```python
from build123d import *

# Parameters (mm, degrees)
HOLE_D             = 4.5
HOLE_DEPTH         = 25
HOLE_CSINK_D       = 9.5
HOLE_CSINK_ANGLE   = 90
POLARPATTERN_COUNT = 6
SKETCH002_W        = 110
SKETCH002_H        = 70.917771
POCKET_DEPTH       = 41.103131
POCKET_DEPTH_BACK  = -41.103131


with BuildPart() as part:
    # Sketch → Revolution (revolve)
    with BuildSketch(Plane.XZ):
        Polygon((-27.5, 18), (-27.5, 0), (-25.5, 0), (-25.5, 40), (-27.5, 45), (-27.5, 25), (-30.5, 22), (-41.102131, 22), (-41.102131, 18), align=None)
    revolve(axis=Axis((0, 0, 0), (0, 0, 1)))

    # Hole
    with Locations(Plane(origin=(0, 0, 22), x_dir=(-1, 0, 0), z_dir=(0, 0, 1))):
        with Locations((35.5, 0)):
            hole = CounterSinkHole(HOLE_D / 2, HOLE_CSINK_D / 2, depth=HOLE_DEPTH, counter_sink_angle=HOLE_CSINK_ANGLE)

    # PolarPattern: Hole ×6 about axis
    polarpattern_axis = Axis((0, 0, 22), (0, 0, 1))
    for i in range(1, POLARPATTERN_COUNT):
        add(hole.rotate(polarpattern_axis, i * 360 / POLARPATTERN_COUNT), mode=Mode.SUBTRACT)

    # Sketch002 → Pocket (cut, two sides)
    with BuildSketch(Plane.YZ) as pocket_sk:
        with Locations((0, -15.458885)):
            Rectangle(SKETCH002_W, SKETCH002_H)
    extrude(amount=-POCKET_DEPTH, mode=Mode.SUBTRACT)
    extrude(pocket_sk.sketch, amount=-POCKET_DEPTH_BACK, mode=Mode.SUBTRACT)


solid = part.part
```
Work out the finished part from the listing and answer in its coordinate system (mm). A direction names the side the tool comes from. Round coordinates to 2 decimals unless told otherwise and drop trailing zeros. Loops run counter-clockwise (first coordinate to the right, second up) from the corner with the lowest first, then second, coordinate; pieces in that order, holes last. Notation, with made-up numbers: M 3.25,-4 L 60.25,-4 A18 cw 60.25,13 Z; hole C 59,67.25 d1. An arc over 180 degrees is marked long. One line per question, with ' | ' between items.
Q1. Find section A-A, the plane y = 0. Give the vertices of the cut face in (x, z).
Conclusion:
outline: M -41.1,20 L -38.25,20 L -40.25,22 L -41.1,22 Z; M -32.75,20 L -25.5,20 L -25.5,40 L -27.5,45 L -27.5,25 L -30.5,22 L -30.75,22 Z; M 25.5,20 L 32.75,20 L 30.75,22 L 30.5,22 L 27.5,25 L 27.5,45 L 25.5,40 Z; M 38.25,20 L 41.1,20 L 41.1,22 L 40.25,22 Z
Q2. Find section C-C, the plane z = 38.25. Give the vertices of the cut face in (x, y).
Conclusion:
outline: C 0,0 d55; hole C 0,0 d51
Q3. Find section B-B, the plane x = 0. Give the vertices of the cut face in (y, z), then the cut area to 3 significant figures.
Conclusion:
outline: M -41.1,20 L -25.5,20 L -25.5,40 L -27.5,45 L -27.5,25 L -30.5,22 L -41.1,22 Z; M 25.5,20 L 41.1,20 L 41.1,22 L 30.5,22 L 27.5,25 L 27.5,45 L 25.5,40 Z | area: 153 mm2
Q4. Consider line 1 along X through (y, z) = (0, 34); line 2 along Y through (x, z) = (-8.5, 25.75). Determine where each line is inside the solid, lowest interval first. Write a range as from..to.
Conclusion:
line 1: x = -27.5..-25.5, 25.5..27.5 | line 2: y = -26.15..-24.04, 24.04..26.15
Q5. A tool of negligible diameter and unlimited length cuts with its end or side. For faces 1 (the flat face through (-18, -19, 20)), 2 (the cylindrical face through (5.961, 26.846, 34.86)), from which of +Z, -Z, +X, -X, +Y, -Y can it reach the whole face along a straight path? Write none if from no direction.
Conclusion:
face 1: -Z, +X, -X, +Y, -Y | face 2: +Z
Q6. Each of these flat-tipped pins is pushed along its axis until it touches: pin 1 Ø12 at (x, z) = (29.5, 36.5) entering from -Y; pin 2 Ø1 at (y, z) = (23.5, 31) entering from +X; pin 3 Ø1.5 at (y, z) = (-21, 23.5) entering from +X. Where does it stop, or does it pass through?
Conclusion:
pin 1: stops at y = -14.28 | pin 2: stops at x = 15.07 | pin 3: stops at x = 21.3
Q7. Find section D-D, the plane x = -35.5. Give the vertices of the cut face in (y, z), then the cut area to 3 significant figures.
Conclusion:
outline: M -20.72,20 L -2.75,20 L -4.75,22 L -20.72,22 Z; M 2.75,20 L 20.72,20 L 20.72,22 L 4.75,22 Z | area: 67.9 mm2
Q8. The mould has two halves that part along X. Classify faces 3 (the conical face through (5.6, 25, 40.3)), 4 (the flat face through (-6.3, 30.3, 22)), 5 (the cylindrical face through (-39.204, -12.346, 20.986)): +X half, -X half, draft (parallel to the pull), parting line (faces both ways), or undercut.
Conclusion:
face 3: undercut | face 4: draft | face 5: parting line
